The listing builds one solid part. Answer for the finished solid, in the listing's coordinates (mm). A direction names the side the tool comes from. Coordinates: 2 decimals unless noted, no trailing zeros. Order: outer loops, then holes, each group sorted by start corner. A loop starts at its lowest first (then second) coordinate and runs counter-clockwise, first axis right, second up. Notation, with made-up numbers: (-40, 70) -> (11, 70) arc R18 cw to (11, 90) -> close; hole circle Ø2 at (5.25, -20.75). An arc over 180 degrees is marked (long way). Return JSON: item names as keys, results as strings.
Autodesk Inventor part; units mm, degrees
ref_plane "YZ Plane" through (0, 0, 0) normal (1, 0, 0) x (0, 1, 0)
ref_plane "XZ Plane" through (0, 0, 0) normal (0, 1, 0) x (-1, 0, 0)
ref_plane "XY Plane" through (0, 0, 0) normal (0, 0, 1) x (1, 0, 0)
sketch "Sketch1" plane through (0, 0, 0) normal (0, 0, 1) x (1, 0, 0)
  line L0 (14.8597, 70) -> (-9.1403, 64)
  line L1 (59.8597, 68) -> (62.8597, 68)
  line L2 (62.8597, 68) -> (62.8597, 51)
  line L3 (62.8597, 17) -> (59.8597, 17)
  line L4 (59.8597, 51) -> (62.8597, 51)
  line L5 (62.8597, 34) -> (62.8597, 17)
  line L6 (-54.1403, 22) -> (-57.1403, 22)
  line L7 (-57.1403, 22) -> (-57.1403, 11)
  line L8 (-57.1403, 11) -> (-54.1403, 11)
  line L9 (-54.1403, 44) -> (-57.1403, 44)
  line L10 (-57.1403, 44) -> (-57.1403, 33)
  line L11 (-57.1403, 33) -> (-54.1403, 33)
  line L12 (-8.5403, 0) -> (-8.5403, -3)
  line L13 (-8.5403, -3) -> (-31.3403, -3)
  line L14 (-31.3403, -3) -> (-31.3403, 0)
  line L15 (32.3597, 0) -> (37.0597, 0)
  line L16 (37.0597, 0) -> (37.0597, -3)
  line L17 (37.0597, -3) -> (14.2597, -3)
  line L18 (14.2597, -3) -> (14.2597, 0)
  line L19 (14.8597, 70) -> (15.5873, 67.0896)
  line L20 (-9.1403, 64) -> (-8.4127, 61.0896)
  line L21 (-54.1403, 22) -> (-54.1403, 33)
  line L22 (59.8597, 17) -> (59.8597, 0)
  line L23 (59.8597, 78.1577) -> (59.8597, 68)
  line L24 (59.8597, 34) -> (59.8597, 51)
  line L25 (-54.1403, 0) -> (-31.3403, 0)
  line L26 (-8.5403, 0) -> (14.2597, 0)
  line L27 (37.0597, 0) -> (59.8597, 0)
  line L28 (-54.1403, 49.6577) -> (-54.1403, 44)
  line L29 (-54.1403, 33) -> (-54.1403, 22)
  line L30 (-54.1403, 33) -> (-54.1403, 22)
  line L31 (-54.1403, 11) -> (-54.1403, 0)
  line L32 (14.8597, 70) -> (-57.1403, 52) construction
  line L33 (-57.1403, 44) -> (-57.1403, 60) construction
  line L34 (-54.1403, 49.6577) -> (-8.4127, 61.0896)
  line L35 (15.5873, 67.0896) -> (59.8597, 78.1577)
  line L36 (59.8597, 34) -> (62.8597, 34)
  line L37 (14.8597, 70) -> (98.136, 90.8191) construction
  line L38 (62.8597, 68) -> (62.8597, 104.4948) construction
  point P0 (0, 0)
  point P1 (62.8597, 82)
  dimension "d3" = 11
  dimension "d4" = 0
  dimension "d5" = 55
  dimension "d6" = 3
  dimension "d8" = 8.5403
  dimension "d9" = 22.8
  dimension "d10" = 3
  dimension "d11" = 3
  dimension "d12" = 114
  dimension "d13" = 24.7386
  dimension "d14" = 3
  dimension "d17" = 17
  dimension "d20" = 22.8
  dimension "d21" = 22.8
  dimension "d22" = 22.8
  dimension "d23" = 82
  dimension "d24" = 48
  dimension "d25" = 48
  dimension "d26" = 17
  dimension "d27" = 11
extrude "Extrusion1" add sketch "Sketch1" along normal blind 3
equation "\"d6\" = tt"
equation "\"d9\" = -0.4 * tt + 0.2 * ht + 2 * tol"
equation "\"d10\" = tt"
equation "\"d11\" = tt"
equation "\"d12\" = -2 * tt + ht"
equation "\"d13\" = 0.2 * d"
equation "\"d14\" = tt"
equation "\"d18\" = tt"
equation "\"d0\" = tt"
equation "\"tt\" = 3"
equation "\"tol\" = 0"
equation "\"tiroir\" = 1"
equation "\"nHoles\" = 4"
equation "\"shelfH\" = 35"
properties part number "glass_separator"
Item 1: The part is cut by section B-B on y = 41.5. Determine the outline of the cut face in (x, z).
Answer list:
{"outline": "(-57.14, 0) -> (59.86, 0) -> (59.86, 3) -> (-57.14, 3) -> close"}
Item 2: The part is cut by section C-C on x = 32. Determine the outline of the cut face in (y, z), plus the area to 3 significant figures.
Answer list:
{"outline": "(-3, 0) -> (71.19, 0) -> (71.19, 3) -> (-3, 3) -> close", "area": "223 mm2"}
Item 3: Flat-ended cylindrical pins translate along their axes: pin 1 (1.5 mm diameter, centred on x = 8.5, z = 1, fed in from -Y); pin 2 (0.9 mm diameter, centred on y = -1.5, z = 1.5, fed in from -X); pin 3 (1.5 mm diameter, centred on x = -56.5, z = 1, fed in from -Y). Find the tip coordinate at first contact, or state that the pin passes through.
Answer list:
{"pin 1": "y = 0", "pin 2": "x = -31.34", "pin 3": "y = 11"}
Item 4: Which of the six approach directions +Z, -Z, +X, -X, +Y, -Y give full straight-line access (tool end or side, diameter ignored) to faces 1 (the flat face through (-56, 33, 1)), 2 (the flat face through (-56, 44, 1)), 3 (the flat face through (37.06, -1, 1)), 4 (the flat face through (37.414, 72.546, 1.479)), 5 (the flat face through (61, 68, 1))?
Answer list:
{"face 1": "+Z, -Z, -X", "face 2": "+Z, -Z, -X, +Y", "face 3": "+Z, -Z, +X, -Y", "face 4": "+Z, -Z, +Y", "face 5": "+Z, -Z, +X, +Y"}
Item 5: Determine the mould class of faces 6 (the flat face through (-54.14, 6, 1)), 7 (the flat face through (48, 0, 1)), 8 (the flat face through (-8.54, -1, 1)), 9 (the flat face through (3, 0, 1)) for opening direction X: pulls with the +X half, pulls with the -X half, needs draft (parallel to the pull), parting line crosses it, or undercut.
Answer list:
{"face 6": "pulls with the -X half", "face 7": "needs draft", "face 8": "undercut", "face 9": "undercut"}
Item 6: Find the intervals of material crossed by probe 1 along X at (y, z) = (46, 0.95); probe 2 along X at (y, z) = (40, 0.7); probe 3 along Y at (x, z) = (12.5, 0.15), in increasing order.
Answer list:
{"probe 1": "-54.14 to 59.86", "probe 2": "-57.14 to 59.86", "probe 3": "0 to 69.41"}
